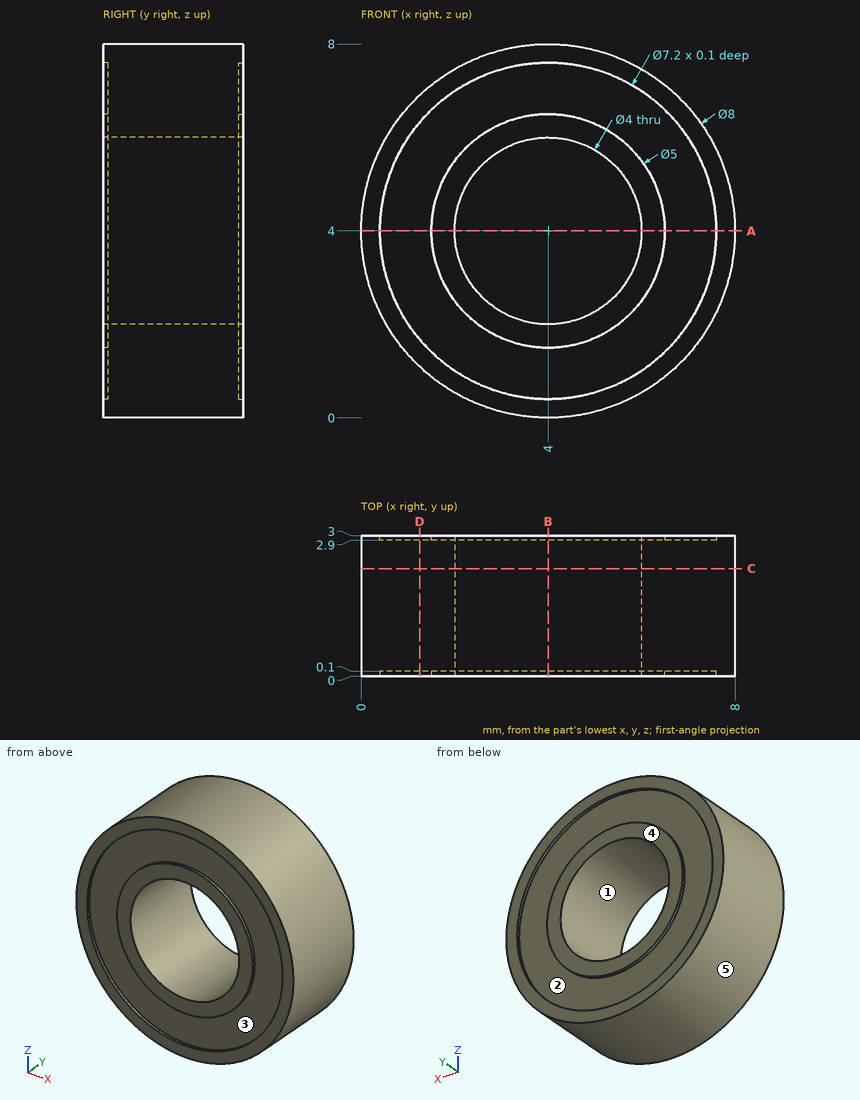
Part print with two shaded views. Sizes in mm from the minimum x, y, z corner. A direction names the side the tool comes from. Coordinates: 2 decimals unless noted, no trailing zeros. Write each loop counter-clockwise with the first axis right and the second up, starting at its lowest first coordinate (ties: lowest second). Pieces come first, ordered by that corner, then holes.
(1) 3-axis set-ups, long thin cutter, end or side, ignore diameter. For the marked faces 1 and 2: which of +Z, -Z, +X, -X, +Y, -Y reach the whole face in a straight line?
(2) Cut at D-D on x = 1.25. List the corners of the cut face in (y, z).
(3) Mould opens along X. For the marked faces 3, 4 and 5 say: pulls with the +X half, pulls with the -X half, needs draft (parallel to the pull), parting line crosses it, or undercut.
(4) Cut at A-A on z = 4. List the corners of the cut face in (x, y), and give its area (3 significant figures).
(5) Drill centre lines: line 1 (Z direction, x = 4, y = 2.95); line 2 (Z direction, x = 4, y = 2.1); line 3 (Z direction, x = 4.5, y = 2.95). Where is each one in solid material? Low to high.
(6) Cut at C-C on y = 2.3. List the corners of the cut face in (x, z).
(7) Pin check, flat tip, straight feed: pin 1 Ø1.5 at (x, y) = (5, 2) entering from +Z. Stop position of the tip, or through.
(8) Cut at B-B on x = 4. List the corners of the cut face in (y, z).
Working result:
1. face 1: +Y, -Y
1. face 2: +Y
2. outline: (0, 1.1) - (3, 1.1) - (3, 1.68) - (2.9, 1.68) - (2.9, 6.32) - (3, 6.32) - (3, 6.9) - (0, 6.9) - (0, 6.32) - (0.1, 6.32) - (0.1, 1.68) - (0, 1.68) - close
3. face 3: undercut
3. face 4: needs draft
3. face 5: parting line crosses it
4. outline: (0, 0) - (0.4, 0) - (0.4, 0.1) - (1.5, 0.1) - (1.5, 0) - (2, 0) - (2, 3) - (1.5, 3) - (1.5, 2.9) - (0.4, 2.9) - (0.4, 3) - (0, 3) - close; (6, 0) - (6.5, 0) - (6.5, 0.1) - (7.6, 0.1) - (7.6, 0) - (8, 0) - (8, 3) - (7.6, 3) - (7.6, 2.9) - (6.5, 2.9) - (6.5, 3) - (6, 3) - close
4. area: 11.6 mm2
5. line 1: z = 0 to 0.4, 1.5 to 2, 6 to 6.5, 7.6 to 8
5. line 2: z = 0 to 2, 6 to 8
5. line 3: z = 0.03 to 0.43, 1.55 to 2.06, 5.94 to 6.45, 7.57 to 7.97
6. outline: circle Ø8 at (4, 4); hole circle Ø4 at (4, 4)
7. pin 1: stops at z = 7.99
8. outline: (0, 0) - (3, 0) - (3, 0.4) - (2.9, 0.4) - (2.9, 1.5) - (3, 1.5) - (3, 2) - (0, 2) - (0, 1.5) - (0.1, 1.5) - (0.1, 0.4) - (0, 0.4) - close; (0, 6) - (3, 6) - (3, 6.5) - (2.9, 6.5) - (2.9, 7.6) - (3, 7.6) - (3, 8) - (0, 8) - (0, 7.6) - (0.1, 7.6) - (0.1, 6.5) - (0, 6.5) - close
